Verification items for the finished model (mm, model axes). Round coordinates to 2 decimals unless told otherwise and drop trailing zeros. Order: outer loops, then holes, each group sorted by start corner. A loop starts at its lowest first (then second) coordinate and runs counter-clockwise, first axis right, second up. Notation, with made-up numbers: (79, 23) -> (111, 23) arc R19 cw to (111, 59) -> close; hole circle Ø5 at (33.5, 31.5). An arc over 180 degrees is marked (long way). Return JSON: item names as keys, results as strings. Group by question number.
1) Section check C-C on x = 25. Enter the section's corners in (y, z), plus the area to 3 significant figures.
2) Draft check along Z on faces 1 (the cylindrical face through (33.05, 1.52, -30.7)), 2 (the flat face through (42, 0, -24)), 3 (the flat face through (36, 1, 0)). Enter one of: pulls with the +Z half, pulls with the -Z half, needs draft (parallel to the pull), parting line crosses it, or undercut.
3) Section check A-A on x = 60. State how many separate pieces and enclosed holes the cut face has, plus the area to 3 significant figures.
4) Depth check by flat-ended pin: pin 1 (6.5 mm diameter, centred on x = 44, z = -44, fed in from +Y). Enter the tip coordinate at first touch or a pass-through.
5) Scan lines: L1, parallel to X at y = 1.8, z = -14.5; L2, parallel to X at y = 1.25, z = -25.5; L3, parallel to Z at x = 25, y = 2.4. Record each from-to range of solid material in increasing order.
Autodesk Inventor part; units mm, degrees
ref_plane "YZ Plane" through (0, 0, 0) normal (1, 0, 0) x (0, 1, 0)
ref_plane "XZ Plane" through (0, 0, 0) normal (0, 1, 0) x (-1, 0, 0)
ref_plane "XY Plane" through (0, 0, 0) normal (0, 0, 1) x (1, 0, 0)
sketch "Sketch1" plane through (0, 0, 0) normal (0, 1, 0) x (-1, 0, 0)
  line L0 (0, 0) -> (-72, 0)
  line L1 (-72, 0) -> (-72, -56)
  line L2 (-72, -56) -> (0, -56)
  line L3 (0, -56) -> (0, 0)
extrude "Extrusion1" add sketch "Sketch1" along normal blind 3
sketch "Sketch2" plane through (0, 3, 0) normal (0, 1, 0) x (1, 0, 0)
  circle A0 centre (12, 44) radius 4
  line L0 (0, 56) -> (0, 0)
  line L1 (72, 56) -> (0, 56)
  circle A1 centre (12, 28) radius 4
  circle A2 centre (12, 12) radius 4
  circle A3 centre (28, 44) radius 4
  circle A4 centre (28, 12) radius 4
  circle A5 centre (44, 44) radius 4
  circle A6 centre (44, 12) radius 4
  circle A7 centre (60, 44) radius 4
  circle A8 centre (60, 12) radius 4
  circle A9 centre (60, 28) radius 4
  circle A10 centre (36, 28) radius 4
  circle A11 centre (4, 52) radius 2
  circle A12 centre (12, 52) radius 2
  circle A13 centre (20, 52) radius 2
  circle A14 centre (28, 52) radius 2
  circle A15 centre (36, 52) radius 2
  circle A16 centre (44, 52) radius 2
  circle A17 centre (52, 52) radius 2
  circle A18 centre (60, 52) radius 2
  circle A19 centre (68, 52) radius 2
  circle A20 centre (4, 44) radius 2
  circle A21 centre (4, 36) radius 2
  circle A22 centre (4, 28) radius 2
  circle A23 centre (4, 20) radius 2
  circle A24 centre (4, 12) radius 2
  circle A25 centre (4, 4) radius 2
  circle A26 centre (12, 4) radius 2
  circle A27 centre (20, 4) radius 2
  circle A28 centre (28, 4) radius 2
  circle A29 centre (36, 4) radius 2
  circle A30 centre (44, 4) radius 2
  circle A31 centre (52, 4) radius 2
  circle A32 centre (60, 4) radius 2
  circle A33 centre (68, 4) radius 2
  circle A34 centre (68, 44) radius 2
  circle A35 centre (68, 36) radius 2
  circle A36 centre (68, 28) radius 2
  circle A37 centre (68, 20) radius 2
  circle A38 centre (68, 12) radius 2
  circle A39 centre (68, 4) radius 2
  circle A40 centre (12, 36) radius 2
  circle A41 centre (20, 36) radius 2
  circle A42 centre (28, 36) radius 2
  circle A43 centre (36, 36) radius 2
  circle A44 centre (44, 36) radius 2
  circle A45 centre (52, 36) radius 2
  circle A46 centre (60, 36) radius 2
  circle A47 centre (12, 20) radius 2
  circle A48 centre (20, 20) radius 2
  circle A49 centre (28, 20) radius 2
  circle A50 centre (36, 20) radius 2
  circle A51 centre (44, 20) radius 2
  circle A52 centre (52, 20) radius 2
  circle A53 centre (60, 20) radius 2
  circle A54 centre (20, 44) radius 2
  circle A55 centre (36, 44) radius 2
  circle A56 centre (52, 44) radius 2
  circle A57 centre (20, 12) radius 2
  circle A58 centre (36, 12) radius 2
  circle A59 centre (52, 12) radius 2
  circle A60 centre (20, 28) radius 2
  circle A61 centre (28, 28) radius 2
  circle A62 centre (44, 28) radius 2
  circle A63 centre (52, 28) radius 2
  dimension "d2" = 8
  dimension "d3" = 8
  dimension "d4" = 8
  dimension "d7" = 16
  dimension "d14" = 16
  dimension "d21" = 16
  dimension "d28" = 24
  dimension "d33" = 4
  dimension "d34" = 2
  dimension "d35" = 2
  dimension "d38" = 8
  dimension "d45" = 8
  dimension "d52" = 8
  dimension "d59" = 8
  dimension "d66" = 8
  dimension "d73" = 8
  dimension "d80" = 8
  dimension "d87" = 8
  dimension "d94" = 8
fillet "Fillet1" radius 1 4 edges at (72, 1.5, -56) (72, 1.5, 0) (0, 1.5, 0) (0, 1.5, -56)
extrude "Extrusion2" cut sketch "Sketch2" against normal blind 4
properties part number "Aluminum Plate"
Check result:
{
 "1": {"outline": "(0, -56) -> (3, -56) -> (3, -46.65) -> (0, -46.65) -> close; (0, -41.35) -> (3, -41.35) -> (3, -14.65) -> (0, -14.65) -> close; (0, -9.35) -> (3, -9.35) -> (3, 0) -> (0, 0) -> close", "area": "136 mm^2"},
 "2": {"face 1": "undercut", "face 2": "needs draft", "face 3": "pulls with the +Z half"},
 "3": {"separate pieces": "8", "enclosed holes": "0", "area": "48.0 mm^2"},
 "4": {"pin 1": "through"},
 "5": {"L1": "0 to 8.88, 15.12 to 24.88, 31.12 to 40.88, 47.12 to 56.88, 63.12 to 72", "L2": "0 to 8.88, 15.12 to 32.88, 39.12 to 56.88, 63.12 to 72", "L3": "-56 to -46.65, -41.35 to -14.65, -9.35 to 0"}
}
